The listing builds one solid part. Answer for the finished solid, in the listing's coordinates (mm). Face numbers are marked on the shaded views. A direction names the side the tool comes from. Round coordinates to 2 decimals unless told otherwise and drop trailing zeros. Write each loop counter-clockwise with the first axis right and the second up, starting at its lowest first coordinate (ties: lowest second). Pieces come first, ordered by that corner, then holes.
Item 1: Find section A-A on x = 9. Give the vertices of the cut face in (y, z).
Item 2: A tool of negligible diameter and unlimited length cuts with its end or side. For the marked faces 1, 2 and 3, from which of +Z, -Z, +X, -X, +Y, -Y can it reach the whole face along a straight path? Write none if from no direction.
Item 3: For a pull along Y with two mould halves and no side action, classify the marked faces 4, 5 and 6 as +Y half, -Y half, draft (parallel to the pull), parting line (faces both ways), or undercut.
Item 4: Each of these flat-tipped pins is pushed along its axis until it touches: pin 1 (4 mm diameter, centred on x = 2, z = 0.5, fed in from +Y); pin 2 (0.7 mm diameter, centred on y = -2, z = -1.5, fed in from -X); pin 3 (6 mm diameter, centred on x = 3, y = 4.5, fed in from +Z); pin 4 (1.5 mm diameter, centred on x = 8.5, z = -1.5, fed in from +Y). Where does it stop, or does it pass through?
Item 5: Find the intervals of material crossed by probe 1 along Y at (x, z) = (7, -0.25); probe 2 along X at (y, z) = (-4, 3.5); probe 3 along Z at (x, y) = (2, 5.5), in increasing order.
Item 6: Find section B-B on x = 5. Give the vertices of the cut face in (y, z), then the cut area to 3 significant figures.
```python
from build123d import *

# Parameters (mm, degrees)
SKETCH1_R           = 6.5
BASEHEAD_DEPTH      = 8
SKETCH2_R           = 4
BASEBODY_DEPTH      = 12
HEXAGONSOCKET_DEPTH = 4
TOPFILLET_R         = 1
CHAMFER1_SIZE       = 0.4


with BuildPart() as part:
    # Sketch1 → BaseHead (new body)
    with BuildSketch(Plane(origin=(0, 0, 0), x_dir=(0, 0, -1), z_dir=(1, 0, 0))):
        Circle(SKETCH1_R)
    extrude(amount=BASEHEAD_DEPTH)

    # Sketch2 → BaseBody (add)
    with BuildSketch(Plane(origin=(8, 0, 0), x_dir=(0, 0, -1), z_dir=(1, 0, 0))):
        Circle(SKETCH2_R)
    extrude(amount=BASEBODY_DEPTH)

    # Sketch3 → HexagonSocket (cut)
    with BuildSketch(Plane(origin=(0, 0, 0), x_dir=(0, 0, -1), z_dir=(1, 0, 0))):
        Polygon((3.464101615, 0), (1.732050808, 3), (-1.732050808, 3), (-3.464101615, 0), (-1.732050808, -3), (1.732050808, -3), align=None)
    extrude(amount=HEXAGONSOCKET_DEPTH, mode=Mode.SUBTRACT)

    # Sketch4 → Cut-Revolve1 (revolve, cut)
    with BuildSketch(Plane(origin=(-4.19613823, 0.75, 0), x_dir=(-1, 0, 0), z_dir=(0, 0, 1)), mode=Mode.PRIVATE) as cut_revolve1_sk:
        Polygon((-8.19613823, 3.75), (-9.928189037, 0.75), (-8.19613823, 0.75), align=None)
    revolve(cut_revolve1_sk.sketch.rotate(Axis((0.838992387, 0, 0), (-1, 0, 0)), 90), axis=Axis((0.838992387, 0, 0), (-1, 0, 0)), mode=Mode.SUBTRACT)

    # TopFillet
    topfillet_edges = [part.edges().sort_by_distance(p)[0] for p in [
        (0, 0, 6.5),
    ]]
    fillet(topfillet_edges, radius=TOPFILLET_R)

    # Chamfer1
    chamfer1_edges = [part.edges().sort_by_distance(p)[0] for p in [
        (20, 0, 4),
    ]]
    chamfer(chamfer1_edges, length=CHAMFER1_SIZE)


solid = part.part
```
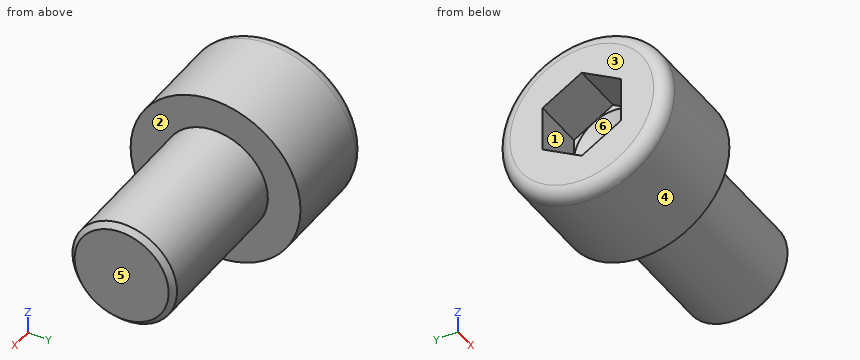
Check values:
1. outline: circle Ø8 at (0, 0)
2. face 1: -X
2. face 2: +X
2. face 3: +Z, -Z, -X, +Y, -Y
3. face 4: parting line
3. face 5: draft
3. face 6: undercut
4. pin 1: stops at y = 6.5
4. pin 2: stops at x = 4.09
4. pin 3: stops at z = 6.32
4. pin 4: stops at y = 6.43
5. probe 1: y = -6.5 to 6.5
5. probe 2: x = 0 to 8
5. probe 3: z = -3.46 to 3.46
6. outline: circle Ø13 at (0, 0); hole circle Ø2.54 at (0, 0)
6. area: 128 mm2
